```python
from build123d import *

# Parameters (mm, degrees)
F0_W     = 500
F0_H     = 200
F0_R     = 3
F1_DEPTH = 30
F2_W     = 10
F2_H     = 10
F3_DEPTH = 500
F5_START = -27
F4_W     = 30
F4_H     = 1
F5_DEPTH = 446


with BuildPart() as f1:
    # F0 (on Right) → F1 (new body)
    with BuildSketch(Plane.YZ):
        Rectangle(F0_W, F0_H)
        with Locations((-235, -50)):
            Circle(F0_R, mode=Mode.SUBTRACT)
        with Locations((235, -50)):
            Circle(F0_R, mode=Mode.SUBTRACT)
        with Locations((-235, 0)):
            Circle(F0_R, mode=Mode.SUBTRACT)
        with Locations((-235, 50)):
            Circle(F0_R, mode=Mode.SUBTRACT)
        with Locations((235, 0)):
            Circle(F0_R, mode=Mode.SUBTRACT)
        with Locations((235, 50)):
            Circle(F0_R, mode=Mode.SUBTRACT)
    extrude(amount=F1_DEPTH)

    # F2 (on face) → F3 (join)
    with BuildSketch(Plane.XZ.offset(250)):
        with Locations((15, -105)):
            Rectangle(F2_W, F2_H)
    extrude(amount=-F3_DEPTH)

    # F4 (on face) → F5 (cut)
    with BuildSketch(Plane.XZ.offset(250).offset(F5_START)):
        with Locations((15, -94.5)):
            Rectangle(F4_W, F4_H)
    extrude(amount=-F5_DEPTH, mode=Mode.SUBTRACT)


solid = f1.part
```
Verification items for the finished model (mm, model axes). A direction names the side the tool comes from. Give positions to 0.01 mm unless a question says otherwise; leave off trailing zeros. Loops run counter-clockwise (first coordinate to the right, second up) from the corner with the lowest first, then second, coordinate; pieces in that order, holes last.
1. Thickness scan on line 1 (Z direction, x = 12.25, y = -235); line 2 (Z direction, x = 17, y = -29); line 3 (Y direction, x = 16.75, z = 51.5). Record the ranges inside material, lowest first.
2. Mould release check, pull along Y, two halves, no side actions. Record for faces 1 (the flat face through (15, -3, -94)), 2 (the flat face through (15, -250, -6)), 3 (the flat face through (25, -3, -100)): released by +Y, released by -Y, zero draft, split by the parting line, or undercut.
3. Go/stop test with flat-tipped pins: pin 1 Ø5 at (x, y) = (24, 30) entering from -Z; pin 2 Ø5 at (y, z) = (18.5, -105.5) entering from +X; pin 3 Ø5 at (y, z) = (9.5, -103) entering from -X. Record where each tip stops, or that it passes through.
4. Section check A-A, the plane y = -53.5. Enter the section's corners in (x, z).
5. Set-up check for faces 4 (the flat face through (20, -4, -105)), 5 (the flat face through (5, -3, -100)), 6 (the flat face through (15, -3, -95)): record each of +Z, -Z, +X, -X, +Y, -Y from which the full face is reachable in a straight line by a thin tool's end or side.
Geometry says:
1. line 1: z = -110 to -53, -47 to -3, 3 to 47, 53 to 100
1. line 2: z = -110 to -95, -94 to 100
1. line 3: y = -250 to -237.6, -232.4 to 232.4, 237.6 to 250
2. face 1: undercut
2. face 2: released by -Y
2. face 3: zero draft
3. pin 1: stops at z = -100
3. pin 2: stops at x = 20
3. pin 3: stops at x = 10
4. outline: (0, -100) - (10, -100) - (10, -110) - (20, -110) - (20, -100) - (30, -100) - (30, -95) - (0, -95) - close; (0, -94) - (30, -94) - (30, 100) - (0, 100) - close
5. face 4: -Z, +X, +Y, -Y
5. face 5: -Z, -X, +Y, -Y
5. face 6: +X, -X
